```python
from build123d import *

# Parameters (mm, degrees)
SKETCH_1_R             = 11
EXTRUDE_1_DEPTH        = 157
SKETCH_2_R             = 11
EXTRUDE_2_DEPTH        = 152
PATTERN_LINEAR_1_COUNT = 2
PATTERN_LINEAR_1_PITCH = 152
CHAMFER_3_SIZE         = 21.999
SKETCH_3_R             = 10.9995
EXTRUDE_3_DEPTH        = 55
FILLET_1_R             = 2


with BuildPart() as part:
    # 草图1 → 拉伸1 (new body)
    with BuildSketch(Plane.XY):
        Circle(SKETCH_1_R)
    extrude_1 = extrude(amount=EXTRUDE_1_DEPTH)

    # 草图2 → 拉伸2 (add)
    with BuildSketch(Plane(origin=(0, 0, 0), x_dir=(1, 0, 0), z_dir=(0, 1, 0))):
        with Locations(Location((0, 0, 0), (0, 0, 180))):
            Circle(SKETCH_2_R)
    extrude(amount=EXTRUDE_2_DEPTH)

    # 阵列(线性)1: 拉伸1 ×2
    with Locations(*[(0, i * PATTERN_LINEAR_1_PITCH, 0) for i in range(1, PATTERN_LINEAR_1_COUNT)]):
        add(extrude_1)

    # 倒角3
    # the kernel refuses this chamfer: 21.999 mm, written as the material it adds along each edge
    with BuildSketch(Plane(origin=(67.574454052, 0, 0), x_dir=(0, -0.9996219169112966, 0.027495876610586372), z_dir=(-1, 0, 0))) as chamfer_3_piece_1_section:
        Polygon((CHAMFER_3_SIZE * 0.999621916911, -CHAMFER_3_SIZE * 0.0274958766106), (-CHAMFER_3_SIZE * 0.0274958766106, -CHAMFER_3_SIZE * 0.999621916911), (0, 0), align=None)
    chamfer_3_piece_1 = extrude(amount=135.148908105, mode=Mode.PRIVATE)
    chamfer_3_piece_1 = chamfer_3_piece_1 & Plane(origin=(0, 0, -4.859651136), x_dir=(1, 0, 0), z_dir=(0, 0, -1)) * Cylinder(11, 359, mode=Mode.PRIVATE)
    chamfer_3_piece_1 = chamfer_3_piece_1 & Plane(origin=(0, -4.859651136, 0), x_dir=(-1, 0, 0), z_dir=(0, -1, 0)) * Cylinder(11, 359, mode=Mode.PRIVATE)
    add(chamfer_3_piece_1)
    with BuildSketch(Plane(origin=(-67.574454052, 152, 0), x_dir=(0, -0.027495876610586986, -0.9996219169112966), z_dir=(1, 0, 0))) as chamfer_3_piece_2_section:
        Polygon((CHAMFER_3_SIZE * 0.999621916911, CHAMFER_3_SIZE * 0.0274958766106), (-CHAMFER_3_SIZE * 0.0274958766106, CHAMFER_3_SIZE * 0.999621916911), (0, 0), align=None)
    chamfer_3_piece_2 = extrude(amount=135.148908105, mode=Mode.PRIVATE)
    chamfer_3_piece_2 = chamfer_3_piece_2 & Plane(origin=(0, 156.859651136, 0), x_dir=(-1, 0, 0), z_dir=(0, -1, 0)) * Cylinder(11, 359, mode=Mode.PRIVATE)
    chamfer_3_piece_2 = chamfer_3_piece_2 & Plane(origin=(0, 152, -4.859651136), x_dir=(1, 0, 0), z_dir=(0, 0, -1)) * Cylinder(11, 359, mode=Mode.PRIVATE)
    add(chamfer_3_piece_2)

    # 草图3 → 拉伸3 (add)
    with BuildSketch(Plane.XY.offset(157)):
        with Locations((0, 152)):
            Circle(SKETCH_3_R)
        Circle(SKETCH_3_R)
    extrude(amount=EXTRUDE_3_DEPTH)

    # 圆角1
    fillet_1_edges = [part.edges().sort_by_distance(p)[0] for p in [
        (-10.9995, 152, 212),
        (-10.9995, 0, 212),
    ]]
    fillet(fillet_1_edges, radius=FILLET_1_R)


solid = part.part
```
The listing builds one solid part. Answer for the finished solid, in the listing's coordinates (mm). A direction names the side the tool comes from. Round coordinates to 2 decimals unless told otherwise and drop trailing zeros. Write each loop counter-clockwise with the first axis right and the second up, starting at its lowest first coordinate (ties: lowest second). Pieces come first, ordered by that corner, then holes. Notation, with made-up numbers: (27, 21.5) -> (81, 21.5) arc R18 cw to (81, 45.5) -> close; hole circle Ø7 at (59.25, 38). An arc over 180 degrees is marked (long way). Write item = value, one per line.
1) Section A-A on z = 161.5 is taken. Write down the section's boundary in (x, y).
Check values:
outline = circle Ø22 at (0, 0); circle Ø22 at (0, 152)
2) Given pin 1 (1 mm diameter, centred on x = -7.5, z = 136.5, fed in from +Y); pin 2 (6 mm diameter, centred on x = -6.5, y = 63, fed in from +Z); pin 3 (3 mm diameter, centred on x = 2.5, z = 170.5, fed in from -Y), each flat-ended and moving along its own axis, determine where each tip first touches the part or whether it passes through.
Check values:
pin_1 = 160.49
pin_2 = 10.43
pin_3 = -10.95
3) Straight lines are drawn through the part: line 1 along Y through (x, z) = (-6.25, 157); line 2 along Y through (x, z) = (1, 81.5); line 3 along Z through (x, y) = (6.25, 146). For each, find the intervals that lie inside material, in ascending order. Write a range as [from, to].
Check values:
line_1 = [-9.05, 9.05], [142.95, 161.05]
line_2 = [-10.95, 10.95], [141.05, 162.95]
line_3 = [-9.05, 212]
4) For a pull along Y with two mould halves and no side action, classify faces 3 (the cylindrical face through (2.38, 74.78, -10.74)), 4 (the flat face through (0, 0, 212)) as released by +Y, released by -Y, zero draft, split by the parting line, or undercut.
Check values:
face_3 = undercut
face_4 = zero draft
5) Which of the six approach directions +Z, -Z, +X, -X, +Y, -Y give full straight-line access (tool end or side, diameter ignored) to faces 1 (the cylindrical face through (5.076, -9.759, 71.824)), 2 (the flat face through (0, 152, 212))?
Check values:
face_1 = +Z
face_2 = +Z, +X, -X, +Y, -Y
6) Section B-B on y = 50 is taken. Write down the section's boundary in (x, z).
Check values:
outline = circle Ø22 at (0, 0)
7) Section C-C on z = 0 is taken. Write down the section's boundary in (x, y).
Check values:
outline = (-11, 0) arc R11 ccw to (11, 0) -> (11, 152) arc R11 ccw to (-11, 152) -> close
